Work out the finished part from the listing and answer in its coordinate system (mm). Face numbers are marked on the shaded views. A direction names the side the tool comes from. Give positions to 0.01 mm unless a question says otherwise; leave off trailing zeros. Write each loop counter-clockwise with the first axis right and the second up, starting at its lowest first coordinate (ties: lowest second). Pieces come first, ordered by that corner, then holes. Notation, with made-up numbers: (-9.5, 37) - (2.5, 37) arc R29 cw to (2.5, 66) - close; hole circle Ø1 at (55, -32.75). An arc over 180 degrees is marked (long way). Write item = value, one per line.
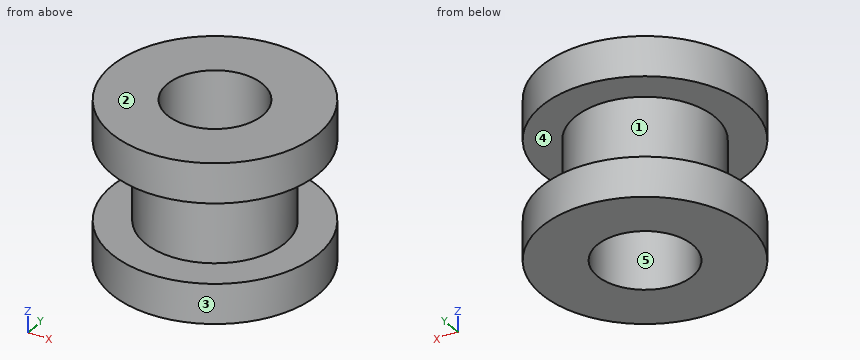
from build123d import *

# Parameters (mm, degrees)
F0_R     = 2.2
F0_R_2   = 1.5
F1_DEPTH = 1.25
F2_R     = 3.25
F2_R_2   = 1.5
F3_DEPTH = 1.25


with BuildPart() as f1:
    # F0 (on Top) → F1 (new body)
    with BuildSketch(Plane.XY):
        Circle(F0_R)
        Circle(F0_R_2, mode=Mode.SUBTRACT)
    extrude(amount=F1_DEPTH)

    # F2 (on face) → F3 (join)
    with BuildSketch(Plane.XY.offset(1.25)):
        Circle(F2_R)
        Circle(F2_R_2, mode=Mode.SUBTRACT)
    extrude(amount=F3_DEPTH)

    # F4: F1 across plane


with BuildPart() as f1_1:
    add(f1.part)
    add(f1.part.mirror(Plane.XY))


solid = f1_1.part
1. For a pull along X with two mould halves and no side action, classify the marked faces 3, 4 and 5 as pulls with the +X half, pulls with the -X half, needs draft (parallel to the pull), parting line crosses it, or undercut.
Solution:
face_3 = parting line crosses it
face_4 = needs draft
face_5 = undercut
2. Find section C-C, the plane z = -0.15. Give the vertices of the cut face in (x, y).
Solution:
outline = circle Ø4.4 at (0, 0); hole circle Ø3 at (0, 0)
3. A tool of negligible diameter and unlimited length cuts with its end or side. For the marked faces 1 and 2, from which of +Z, -Z, +X, -X, +Y, -Y can it reach the whole face along a straight path? Write none if from no direction.
Solution:
face_1 = none
face_2 = +Z, +X, -X, +Y, -Y
4. Given pin 1 (3 mm diameter, centred on y = -2.5, z = 0, fed in from +X), flat-ended and moving along its own axis, determine where the tip first touches the part or whether it passes through.
Solution:
pin_1 = 2.79
5. Find section D-D, the plane x = 1.75. Give the vertices of the cut face in (y, z), then the cut area to 3 significant figures.
Solution:
outline = (-2.74, -2.5) - (2.74, -2.5) - (2.74, -1.25) - (1.33, -1.25) - (1.33, 1.25) - (2.74, 1.25) - (2.74, 2.5) - (-2.74, 2.5) - (-2.74, 1.25) - (-1.33, 1.25) - (-1.33, -1.25) - (-2.74, -1.25) - close
area = 20.4 mm^2
6. Straight lines are drawn through the part: line 1 (Z direction, x = -1.25, y = -2); line 2 (Y direction, x = 0, z = -1.3); line 3 (Y direction, x = 0, z = -0.6). For each, find the intervals that lie inside material, in ascending order.
Solution:
line_1 = -2.5 to -1.25, 1.25 to 2.5
line_2 = -3.25 to -1.5, 1.5 to 3.25
line_3 = -2.2 to -1.5, 1.5 to 2.2
7. Find section A-A, the plane x = 0. Give the vertices of the cut face in (y, z), then the cut area to 4 significant figures.
Solution:
outline = (-3.25, -2.5) - (-1.5, -2.5) - (-1.5, 2.5) - (-3.25, 2.5) - (-3.25, 1.25) - (-2.2, 1.25) - (-2.2, -1.25) - (-3.25, -1.25) - close; (1.5, -2.5) - (3.25, -2.5) - (3.25, -1.25) - (2.2, -1.25) - (2.2, 1.25) - (3.25, 1.25) - (3.25, 2.5) - (1.5, 2.5) - close
area = 12.25 mm^2
